Here's the drawing with two shaded views (mm, measured from the low corner). I have some questions. A direction names the side the tool comes from. Round coordinates to 2 decimals unless told otherwise and drop trailing zeros. Loops run counter-clockwise (first coordinate to the right, second up) from the corner with the lowest first, then second, coordinate; pieces in that order, holes last. Notation, with made-up numbers: (47, -23.75) -> (98, -23.75) arc R22 ccw to (98, -3.75) -> close; hole circle Ø1 at (23.25, 86.25). An arc over 180 degrees is marked (long way). One line per item, written item: value. Start each with the question number.
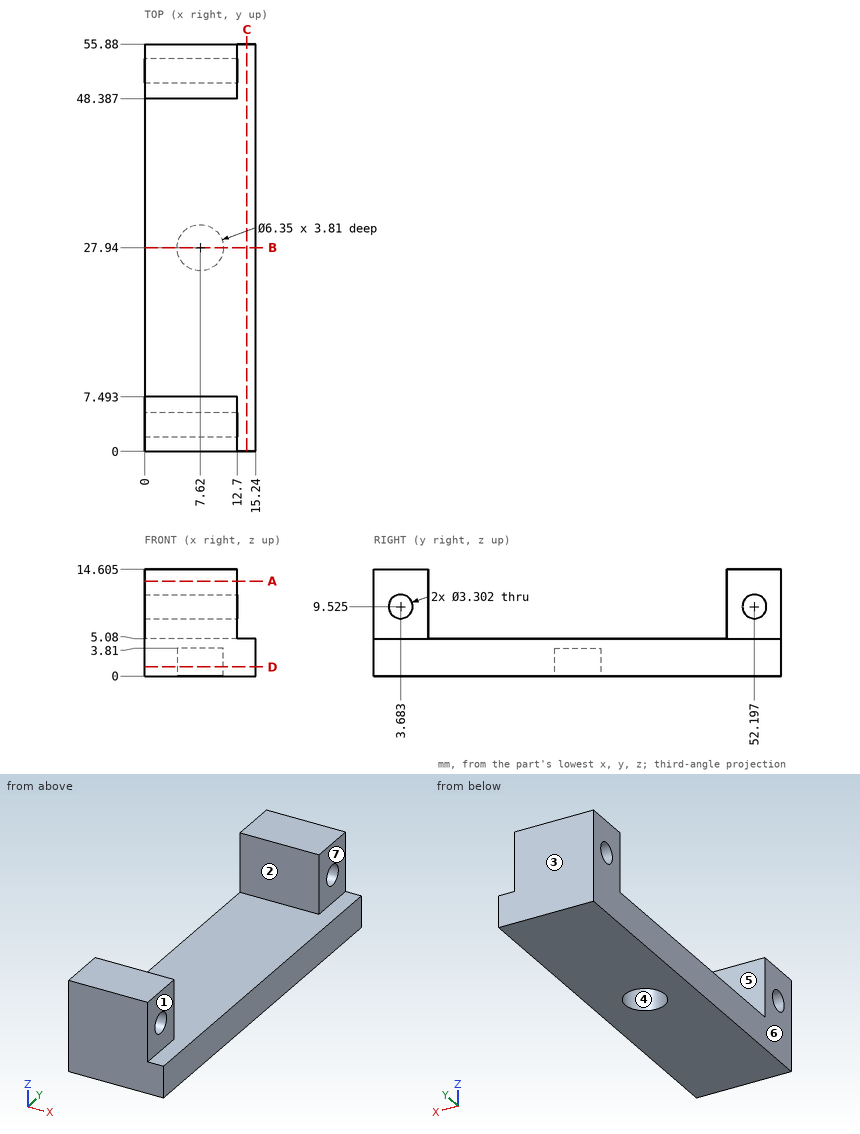
Q1. I want a section at C-C on x = 14. Please give me the cut outline in (y, z), plus the area to 3 significant figures.
Q2. I want a section at B-B on y = 27.94. Please give me the cut outline in (x, z) (3 decimals), plus the area to 3 significant figures.
Q3. Will these pins go through, and if not, where does the flat tip stop? P1, Ø5, axis at x = 8, y = 27, coming from the -Z side; P2, Ø7.5, axis at x = 5, y = 15, coming from the +Z side.
Q4. I want a section at A-A on z = 13. Please give me the cut outline in (x, y).
Q5. I want a section at D-D on z = 1.25. Please give me the cut outline in (x, y) (3 decimals).
Q6. If we mould it in two halves opening along Y, with no side actions, what happens to the marked faces 1, 2, 3 and 4? For each: released by +Y, released by -Y, zero draft, split by the parting line, or undercut.
Q7. If I drill on line 1 along Y through (x, z) = (1, 12); line 2 along X through (y, z) = (27.94, 0.9) (3 decimals); line 3 along Z through (x, y) = (10.25, 8), over which ranges is the centre line in solid material (lowest first)?
Q8. Which directions (+Z, -Z, +X, -X, +Y, -Y) give clear straight access to the entire face, cutting with the end or side of a thin tool? Please do the marked faces 5, 6 and 7.
Answers below:
1. outline: (0, 0) -> (55.88, 0) -> (55.88, 5.08) -> (0, 5.08) -> close
1. area: 284 mm^2
2. outline: (0, 0) -> (4.445, 0) -> (4.445, 3.81) -> (10.795, 3.81) -> (10.795, 0) -> (15.24, 0) -> (15.24, 5.08) -> (0, 5.08) -> close
2. area: 53.2 mm^2
3. P1: stops at z = 0
3. P2: stops at z = 5.08
4. outline: (0, 0) -> (12.7, 0) -> (12.7, 7.49) -> (0, 7.49) -> close; (0, 48.39) -> (12.7, 48.39) -> (12.7, 55.88) -> (0, 55.88) -> close
5. outline: (0, 0) -> (15.24, 0) -> (15.24, 55.88) -> (0, 55.88) -> close; hole circle Ø6.35 at (7.62, 27.94)
6. face 1: zero draft
6. face 2: undercut
6. face 3: released by +Y
6. face 4: undercut
7. line 1: y = 0 to 7.49, 48.39 to 55.88
7. line 2: x = 0 to 4.445, 10.795 to 15.24
7. line 3: z = 0 to 5.08
8. face 5: +Z, +X, -X
8. face 6: +Z, -Z, -X, +Y, -Y
8. face 7: +Z, +X, +Y, -Y
